Check sheet for the modelled part. Datum: model origin and axes. Units: mm. A direction names the side the tool comes from. Coordinates: 2 decimals unless noted, no trailing zeros. Write each loop counter-clockwise with the first axis right and the second up, starting at its lowest first coordinate (ties: lowest second). Pieces come first, ordered by that corner, then holes. Notation, with made-up numbers: M -31.5,-3.75 L 4.5,-3.75 A29 ccw 4.5,25.25 Z; hole C -15,-32.75 d6. An arc over 180 degrees is marked long. Answer as CSV lines item,"result". Start each with the question number.
1) Section check B-B (z = 0). Record the cut outline in (x, y).
2) Section check A-A (x = 0). Record the cut outline in (y, z), and give its area (3 significant figures).
3) Section check D-D (x = 5.5). Record the cut outline in (y, z), and give its area (3 significant figures).
4) Go/stop test with flat-tipped pins: pin 1 Ø5 at (y, z) = (10.5, -3) entering from +X; pin 2 Ø5 at (x, y) = (1.5, 6) entering from -Z; pin 3 Ø2 at (x, y) = (1, 13) entering from +Z. Record where each tip stops, or that it passes through.
5) Section check C-C (y = 1.25). Record the cut outline in (x, z).
6) Access from +Z, -Z, +X, -X, +Y, -Y to the whole of each face (thin tool, end or side, straight path). Record for faces 5 (the cylindrical face through (6.466, 9.084, 2.681)), 6 (the cylindrical face through (-3.2, 7.6, 2.4)).
7) Material ranges on L1, parallel to X at y = 6, z = 0; L2, parallel to Y at x = 5.7, z = 0, recorded low to high. Write a range as [from, to].
8) Draft check along Y on faces 1 (the cylindrical face through (0, 1, -9)), 2 (the flat face through (-0.2, 3, -7.4)), 3 (the flat face through (-5, 0, 0)), 4 (the cylindrical face through (5.38, 8.5, 0.07)). Enter one of: +Y half, -Y half, draft (parallel to the pull), parting line (faces both ways), or undercut.
Autodesk Inventor part; units mm, degrees
ref_plane "Plan de construction1" through (7, 15, 0) normal (1, 0, 0) x (0, 1, 0)
ref_plane "XZ Plane" through (0, 0, 0) normal (0, 1, 0) x (-1, 0, 0)
ref_plane "XY Plane" through (0, 0, 0) normal (0, 0, 1) x (1, 0, 0)
sketch "Esquisse1" plane through (0, 0, 0) normal (0, 1, 0) x (-1, 0, 0)
  circle A0 centre (0, 0) radius 11
  dimension "d0" = 22
extrude "Extrusion1" add sketch "Esquisse1" along normal blind 15
sketch "Esquisse2" plane through (0, 15, 0) normal (0, 1, 0) x (1, 0, 0)
  circle A0 centre (0, 0) radius 11
  circle A1 centre (0, 0) radius 7
  dimension "d3" = 14
extrude "Extrusion2" cut sketch "Esquisse2" against normal blind 12
sketch "Esquisse3" plane through (0, 15, 0) normal (0, 1, 0) x (1, 0, 0)
  circle A0 centre (0, 0) radius 7
  circle A1 centre (0, 0) radius 4
  dimension "d6" = 8
extrude "Extrusion3" cut sketch "Esquisse3" against normal through all contours A1
sketch "Esquisse4" plane through (0, 0, 0) normal (0, -1, 0) x (1, 0, 0)
  circle A0 centre (0, 0) radius 11
  circle A1 centre (0, 11) radius 2
  circle A2 centre (0, -11) radius 2
  dimension "d9" = 4
  dimension "d10" = 4
extrude "Extrusion4" cut sketch "Esquisse4" against normal through all contours A1 A0 | A0 A1 | A2 A0 | A0 A2
ref_plane "Plan de construction1" through (7, 15, 0) normal (1, 0, 0) x (0, 1, 0)
sketch "Esquisse5" plane through (7, 15, 0) normal (1, 0, 0) x (0, 1, 0)
  circle A0 centre (-5, 0) radius 1.5
  line L0 (0, -7) -> (0, 7)
  point P0 (-15, 0)
  dimension "d13" = 3
  dimension "d16" = 5
extrude "Extrusion5" cut sketch "Esquisse5" against normal blind 5
thread "Filetage1"
equation "\"d10\" = d9"
properties part number "Raccord-Mat-Potence" material "Aluminium 6061"
Results found:
1,outline,"M -11,0 L -4,0 L -4,15 L -7,15 L -7,3 L -11,3 Z; M 4,0 L 11,0 L 11,3 L 7,3 L 7,8.5 L 4,8.5 Z; M 4,11.5 L 7,11.5 L 7,15 L 4,15 Z"
2,outline,"M 0,-9 L 3,-9 L 3,-7 L 15,-7 L 15,-4 L 0,-4 Z; M 0,4 L 15,4 L 15,7 L 3,7 L 3,9 L 0,9 Z"
2,area,"102 mm2"
3,outline,"M 0,-9.53 L 3,-9.53 L 3,-4.33 L 15,-4.33 L 15,4.33 L 3,4.33 L 3,9.53 L 0,9.53 Z; hole C 10,0 d3"
3,area,"154 mm2"
4,pin 1,"stops at x = 6.97"
4,pin 2,"stops at z = -7"
4,pin 3,"stops at z = 7"
5,outline,"M -1.99,-10.82 A2 cw 1.99,-10.82 A11 ccw 1.99,10.82 A2 cw -1.99,10.82 A11 ccw Z; hole C 0,0 d8"
6,face 5,"+Y"
6,face 6,"+Y, -Y"
7,L1,"x = [-7, -4], [4, 7]"
7,L2,"y = [0, 8.5], [11.5, 15]"
8,face 1,"draft"
8,face 2,"+Y half"
8,face 3,"-Y half"
8,face 4,"undercut"
